```python
from build123d import *

# Parameters (mm, degrees)
SKETCH1_R                            = 60
BOSS_EXTRUDE1_DEPTH                  = 160
CHAMFER1_SIZE                        = 20
CHAMFER1_SIZE2                       = 30
SHELL2_T                             = -5
SKETCH7_R                            = 15
CUT_EXTRUDE1_DEPTH                   = 7
SKETCH8_R                            = 15
CUT_EXTRUDE2_DEPTH                   = 7
SKETCH9_R                            = 23.5
BOSS_EXTRUDE2_DEPTH                  = 7
BOSS_EXTRUDE2_DIRECTION_2_REACH      = 210.806
BOSS_EXTRUDE2_DIRECTION_2_END_RADIUS = 60
SKETCH10_R                           = 23.5
BOSS_EXTRUDE3_DEPTH                  = 7
BOSS_EXTRUDE3_DIRECTION_2_REACH      = 214.906
BOSS_EXTRUDE3_DIRECTION_2_END_RADIUS = 60
SKETCH12_W                           = 35
SKETCH12_H                           = 40
CUT_EXTRUDE3_DEPTH                   = 32
CUT_EXTRUDE4_REACH                   = 221.026
CUT_EXTRUDE4_END_RADIUS              = 55
SKETCH14_W                           = 3
SKETCH14_H                           = 15
CUT_EXTRUDE5_REACH                   = 218.344
CUT_EXTRUDE5_END_RADIUS              = 55
SKETCH15_W                           = 3
SKETCH15_H                           = 15
CUT_EXTRUDE6_REACH                   = 218.344
CUT_EXTRUDE6_END_RADIUS              = 55
SKETCH16_W                           = 3
SKETCH16_H                           = 15
CUT_EXTRUDE7_REACH                   = 221.026
CUT_EXTRUDE7_END_RADIUS              = 55
SKETCH17_W                           = 3
SKETCH17_H                           = 15
BOSS_EXTRUDE5_REACH                  = 185.546
SKETCH18_R                           = 1.5
BOSS_EXTRUDE5_DIRECTION_2_REACH      = 185.546


with BuildPart() as part:
    # Sketch1 → Boss-Extrude1 (new body)
    with BuildSketch(Plane.XY):
        Circle(SKETCH1_R)
    extrude(amount=BOSS_EXTRUDE1_DEPTH)

    # Chamfer1
    chamfer1_edges = [part.edges().sort_by_distance(p)[0] for p in [
        (-60, 0, 0),
    ]]
    chamfer1_side = [part.faces().sort_by_distance(p)[0] for p in [
        (0, 0, 0),
    ]]
    chamfer(chamfer1_edges, length=CHAMFER1_SIZE, length2=CHAMFER1_SIZE2, reference=chamfer1_side[0])

    # Shell2
    shell2_openings = [part.faces().sort_by_distance(p)[0] for p in [
        (0, 0, 160),
        (0, 0, 0),
    ]]
    offset(amount=SHELL2_T, openings=shell2_openings, kind=Kind.INTERSECTION)

    # Sketch7 → Cut-Extrude1 (cut)
    with BuildSketch(Plane(origin=(-30, -51.961524227, 0), x_dir=(-0.866025403784438, 0.5000000000000011, 0), z_dir=(-0.5000000000000011, -0.866025403784438, 0))):
        with Locations(Location((0, -115, 0), (0, 0, 180))):
            Circle(SKETCH7_R)
    extrude(amount=-CUT_EXTRUDE1_DEPTH, mode=Mode.SUBTRACT)

    # Sketch8 → Cut-Extrude2 (cut)
    with BuildSketch(Plane(origin=(30, -51.961524227, 0), x_dir=(-0.8660254037844451, -0.4999999999999888, 0), z_dir=(0.4999999999999888, -0.8660254037844451, 0))):
        with Locations(Location((0, -115, 0), (0, 0, 180))):
            Circle(SKETCH8_R)
    extrude(amount=-CUT_EXTRUDE2_DEPTH, mode=Mode.SUBTRACT)

    # Sketch9 → Boss-Extrude2 (add)
    with BuildSketch(Plane.ZY.offset(60)):
        with Locations((110, 0)):
            Circle(SKETCH9_R)
    extrude(amount=BOSS_EXTRUDE2_DEPTH)

    # Boss-Extrude2 direction 2: up to this cylinder (the profile starts outside it)
    boss_extrude2_direction_2_end = Plane(origin=(0, 0, 110), z_dir=(0, 0, -1)) * Cylinder(BOSS_EXTRUDE2_DIRECTION_2_END_RADIUS, 542.612, mode=Mode.PRIVATE)
    # Sketch9 → Boss-Extrude2 direction 2 (add, up to the surface)
    with BuildSketch(Plane.ZY.offset(60), mode=Mode.PRIVATE) as boss_extrude2_direction_2_sk1:
        with Locations((110, 0)):
            Circle(SKETCH9_R)
    boss_extrude2_direction_2_tool1 = extrude(boss_extrude2_direction_2_sk1.sketch, amount=-BOSS_EXTRUDE2_DIRECTION_2_REACH, mode=Mode.PRIVATE) - boss_extrude2_direction_2_end
    add(boss_extrude2_direction_2_tool1.solids().sort_by_distance((-60, 0, 110))[0])
    add(boss_extrude2_direction_2_tool1.solids().sort_by_distance((-60, 0, 110))[1])

    # Sketch10 → Boss-Extrude3 (add)
    with BuildSketch(Plane(origin=(60, 0, 0), x_dir=(0, 0, -1), z_dir=(1, 0, 0))):
        with Locations(Location((-110, 0, 0), (0, 0, 180))):
            Circle(SKETCH10_R)
    extrude(amount=BOSS_EXTRUDE3_DEPTH)

    # Boss-Extrude3 direction 2: up to this cylinder (the profile starts outside it)
    boss_extrude3_direction_2_end = Plane(origin=(0, 0, 110), z_dir=(0, 0, -1)) * Cylinder(BOSS_EXTRUDE3_DIRECTION_2_END_RADIUS, 550.812, mode=Mode.PRIVATE)
    # Sketch10 → Boss-Extrude3 direction 2 (add, up to the surface)
    with BuildSketch(Plane(origin=(60, 0, 0), x_dir=(0, 0, -1), z_dir=(1, 0, 0)), mode=Mode.PRIVATE) as boss_extrude3_direction_2_sk1:
        with Locations(Location((-110, 0, 0), (0, 0, 180))):
            Circle(SKETCH10_R)
    boss_extrude3_direction_2_tool1 = extrude(boss_extrude3_direction_2_sk1.sketch, amount=-BOSS_EXTRUDE3_DIRECTION_2_REACH, mode=Mode.PRIVATE) - boss_extrude3_direction_2_end
    add(boss_extrude3_direction_2_tool1.solids().sort_by_distance((60, 0, 110))[0])
    add(boss_extrude3_direction_2_tool1.solids().sort_by_distance((60, 0, 110))[1])

    # Sketch12 → Cut-Extrude3 (cut)
    with BuildSketch(Plane(origin=(0, -60, 0), x_dir=(-1, 0, 0), z_dir=(0, -1, 0))):
        with Locations((0, -20)):
            Rectangle(SKETCH12_W, SKETCH12_H)
    extrude(amount=-CUT_EXTRUDE3_DEPTH, mode=Mode.SUBTRACT)

    # Cut-Extrude4: up to this cylinder (the profile starts outside it)
    cut_extrude4_end = Plane(origin=(0, 0, 137), z_dir=(0, 0, -1)) * Cylinder(CUT_EXTRUDE4_END_RADIUS, 553.052, mode=Mode.PRIVATE)
    # Sketch14 → Cut-Extrude4 (cut, up to the surface)
    with BuildSketch(Plane(origin=(38.567256581, -45.962666587, 0), x_dir=(-0.7660444431189859, -0.6427876096865299, 0), z_dir=(0.6427876096865299, -0.7660444431189859, 0)), mode=Mode.PRIVATE) as cut_extrude4_sk1:
        with Locations((0, -137)):
            Rectangle(SKETCH14_W, SKETCH14_H)
    cut_extrude4_tool1 = extrude(cut_extrude4_sk1.sketch, amount=-CUT_EXTRUDE4_REACH, mode=Mode.PRIVATE) - cut_extrude4_end
    add(cut_extrude4_tool1.solids().sort_by_distance((38.567257, -45.962667, 137))[0], mode=Mode.SUBTRACT)

    # Cut-Extrude5: up to this cylinder (the profile starts outside it)
    cut_extrude5_end = Plane(origin=(0, 0, 137), z_dir=(0, 0, -1)) * Cylinder(CUT_EXTRUDE5_END_RADIUS, 547.688, mode=Mode.PRIVATE)
    # Sketch15 → Cut-Extrude5 (cut, up to the surface)
    with BuildSketch(Plane(origin=(20.5212086, -56.381557247, 0), x_dir=(-0.9396926207859128, -0.3420201433256568, 0), z_dir=(0.3420201433256568, -0.9396926207859128, 0)), mode=Mode.PRIVATE) as cut_extrude5_sk1:
        with Locations((0, -137)):
            Rectangle(SKETCH15_W, SKETCH15_H)
    cut_extrude5_tool1 = extrude(cut_extrude5_sk1.sketch, amount=-CUT_EXTRUDE5_REACH, mode=Mode.PRIVATE) - cut_extrude5_end
    add(cut_extrude5_tool1.solids().sort_by_distance((20.521209, -56.381557, 137))[0], mode=Mode.SUBTRACT)

    # Cut-Extrude6: up to this cylinder (the profile starts outside it)
    cut_extrude6_end = Plane(origin=(0, 0, 137), z_dir=(0, 0, -1)) * Cylinder(CUT_EXTRUDE6_END_RADIUS, 547.688, mode=Mode.PRIVATE)
    # Sketch16 → Cut-Extrude6 (cut, up to the surface)
    with BuildSketch(Plane(origin=(-20.5212086, -56.381557247, 0), x_dir=(-0.9396926207859082, 0.3420201433256693, 0), z_dir=(-0.3420201433256693, -0.9396926207859082, 0)), mode=Mode.PRIVATE) as cut_extrude6_sk1:
        with Locations((0, -137)):
            Rectangle(SKETCH16_W, SKETCH16_H)
    cut_extrude6_tool1 = extrude(cut_extrude6_sk1.sketch, amount=-CUT_EXTRUDE6_REACH, mode=Mode.PRIVATE) - cut_extrude6_end
    add(cut_extrude6_tool1.solids().sort_by_distance((-20.521209, -56.381557, 137))[0], mode=Mode.SUBTRACT)

    # Cut-Extrude7: up to this cylinder (the profile starts outside it)
    cut_extrude7_end = Plane(origin=(0, 0, 137), z_dir=(0, 0, -1)) * Cylinder(CUT_EXTRUDE7_END_RADIUS, 553.052, mode=Mode.PRIVATE)
    # Sketch17 → Cut-Extrude7 (cut, up to the surface)
    with BuildSketch(Plane(origin=(-38.567256581, -45.962666587, 0), x_dir=(-0.7660444431189771, 0.6427876096865406, 0), z_dir=(-0.6427876096865405, -0.766044443118977, 0)), mode=Mode.PRIVATE) as cut_extrude7_sk1:
        with Locations((0, -137)):
            Rectangle(SKETCH17_W, SKETCH17_H)
    cut_extrude7_tool1 = extrude(cut_extrude7_sk1.sketch, amount=-CUT_EXTRUDE7_REACH, mode=Mode.PRIVATE) - cut_extrude7_end
    add(cut_extrude7_tool1.solids().sort_by_distance((-38.567257, -45.962667, 137))[0], mode=Mode.SUBTRACT)

    # Boss-Extrude5: up to this cone (the profile starts inside it)
    boss_extrude5_end = Plane(origin=(0, 0, 2.5), z_dir=(0, 0, 1)).offset(-53.486120811) * Cone(1e-06, 183.459690901, 275.189535352, align=(Align.CENTER, Align.CENTER, Align.MIN), mode=Mode.PRIVATE)
    # Sketch18 → Boss-Extrude5 (add, up to the surface)
    with BuildSketch(Plane(origin=(0, 0, 0), x_dir=(0, 0, -1), z_dir=(1, 0, 0)), mode=Mode.PRIVATE) as boss_extrude5_sk1:
        with Locations(Location((-2.5, -10.5, 0), (0, 0, 212.572301633))):
            Circle(SKETCH18_R)
    boss_extrude5_tool1 = extrude(boss_extrude5_sk1.sketch, amount=BOSS_EXTRUDE5_REACH, mode=Mode.PRIVATE) & boss_extrude5_end
    add(boss_extrude5_tool1.solids().sort_by_distance((0, -10.5, 2.5))[0])

    # Boss-Extrude5 direction 2: up to this cone (the profile starts inside it)
    boss_extrude5_direction_2_end = Plane(origin=(0, 0, 2.5), z_dir=(0, 0, 1)).offset(-53.486120811) * Cone(1e-06, 183.459690901, 275.189535352, align=(Align.CENTER, Align.CENTER, Align.MIN), mode=Mode.PRIVATE)
    # Sketch18 → Boss-Extrude5 direction 2 (add, up to the surface)
    with BuildSketch(Plane(origin=(0, 0, 0), x_dir=(0, 0, -1), z_dir=(1, 0, 0)), mode=Mode.PRIVATE) as boss_extrude5_direction_2_sk1:
        with Locations(Location((-2.5, -10.5, 0), (0, 0, 212.572301633))):
            Circle(SKETCH18_R)
    boss_extrude5_direction_2_tool1 = extrude(boss_extrude5_direction_2_sk1.sketch, amount=-BOSS_EXTRUDE5_DIRECTION_2_REACH, mode=Mode.PRIVATE) & boss_extrude5_direction_2_end
    add(boss_extrude5_direction_2_tool1.solids().sort_by_distance((0, -10.5, 2.5))[0])


solid = part.part
```
Check sheet for the modelled part. Datum: model origin and axes. Units: mm. A direction names the side the tool comes from. Round coordinates to 2 decimals unless told otherwise and drop trailing zeros. Order: outer loops, then holes, each group sorted by start corner. A loop starts at its lowest first (then second) coordinate and runs counter-clockwise, first axis right, second up.
1) Scan lines: line 1 (X direction, y = -43.5, z = 134); line 2 (X direction, y = 0, z = 112.5); line 3 (Y direction, x = 0, z = 75). Record each from-to range of solid material in increasing order.
2) Tool access check on faces 5 (the cylindrical face through (-7.16, 54.53, 94.86)), 6 (the flat face through (-17.5, -46, 20)), 7 (the flat face through (-21.08, -53.53, 137.1)), 8 (the flat face through (20, -54, 129.5)). Record the directions out of +Z, -Z, +X, -X, +Y, -Y that give a thin tool (end or side, any length) a straight path to the whole face; none if there is none.
3) Section check B-B (x = 27.5). Give the number of separate pieces and of enclosed holes in the cut face, and give its area (3 significant figures).
4) Section check A-A (z = 110). Record the boundary of the cut face in (x, y), and give its area (3 significant figures).
5) Go/stop test with flat-tipped pins: pin 1 Ø22.5 at (y, z) = (-42.5, 29) entering from +X; pin 2 Ø12 at (x, z) = (3.5, 32) entering from +Y; pin 3 Ø1 at (x, y) = (-48.5, 3) entering from -Z; pin 4 Ø1 at (x, y) = (53.5, 27.5) entering from +Z. Record where each tip stops, or that it passes through.
6) Mould release check, pull along Y, two halves, no side actions. Record for faces 1 (the flat face through (-35.8, -45, 137.1)), 2 (the flat face through (18.26, -54.56, 137.1)), 3 (the flat face through (21.08, -53.53, 137.1)), 4 (the flat face through (0, -57, 40)): +Y half, -Y half, draft (parallel to the pull), parting line (faces both ways), or undercut.
7) Section check C-C (z = 53.5). Record the boundary of the cut face in (x, y).
Result:
1. line 1: x = -41.32 to -38.46, -34.54 to -33.66, 33.66 to 34.54, 38.46 to 41.32
1. line 2: x = -67 to -55, 55 to 67
1. line 3: y = -60 to -55, 55 to 60
2. face 5: +Z
2. face 6: -Z, -Y
2. face 7: -Y
2. face 8: none
3. separate pieces: 4
3. enclosed holes: 0
3. area: 1,770 mm2
4. outline: (-67, -23.5) - (-55.21, -23.5) arc R60 ccw to (-41.4, -43.43) - (-38.82, -38.96) arc R55 cw (long way) to (38.82, -38.96) - (41.4, -43.43) arc R60 ccw to (55.21, -23.5) - (67, -23.5) - (67, 23.5) - (55.21, 23.5) arc R60 ccw to (-55.21, 23.5) - (-67, 23.5) - close; (-16.91, -57.57) arc R60 ccw to (16.91, -57.57) - (14.33, -53.1) arc R55 cw to (-14.33, -53.1) - close
4. area: 2,330 mm2
5. pin 1: stops at x = 51.19
5. pin 2: stops at y = 60
5. pin 3: stops at z = 12.14
5. pin 4: stops at z = 160
6. face 1: undercut
6. face 2: undercut
6. face 3: -Y half
6. face 4: draft
7. outline: circle Ø120 at (0, 0); hole circle Ø110 at (0, 0)
